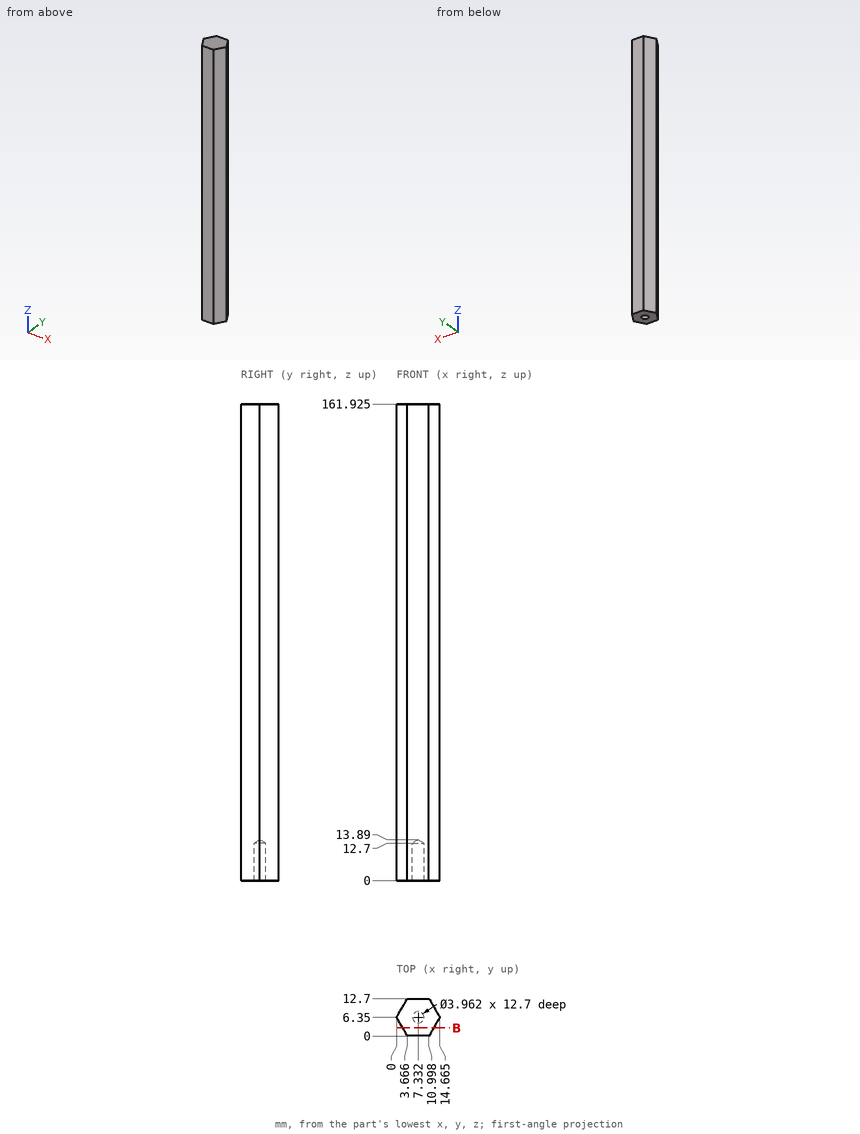
The figure shows three views and two pictorial views of one solid part (mm, origin at its lowest corner). Answer the questions. Give positions to 0.01 mm unless a question says otherwise; leave off trailing zeros. Write each loop counter-clockwise with the first axis right and the second up, starting at its lowest first coordinate (ties: lowest second). Pieces come first, ordered by that corner, then holes. Notation, with made-up numbers: M 21,70.25 L 72,70.25 A25 cw 72,83.25 Z; hole C 4.5,72.5 d5. An arc over 180 degrees is marked long. Write each question's results on one line, items separated by ' | '.
Q1. Flat-ended cylindrical pins translate along their axes: P1, Ø5, axis at y = 7, z = 51.5, coming from the -X side; P2, Ø6, axis at y = 3, z = 106.5, coming from the +X side; P3, Ø1.5, axis at y = 5.5, z = 54.5, coming from the -X side. Find the tip coordinate at first contact, or state that the pin passes through.
Output values:
P1: x = 0 | P2: x = 14.46 | P3: x = 0.06
Q2. Section B-B, the plane y = 2.75 is taken. Write down the section's boundary in (x, z) (1 decimal), then the cut area to 3 significant figures.
Output values:
outline: M 2.1,0 L 12.6,0 L 12.6,161.9 L 2.1,161.9 Z | area: 1,700 mm2
Q3. Consider L1, parallel to Y at x = 11, z = 110 (1 decimal); L2, parallel to X at y = 6, z = 11; L3, parallel to X at y = 0.5, z = 27. Determine where each line is inside the solid, lowest interval first. Write a range as from..to.
Output values:
L1: 0..12.7 | L2: 0.2..5.38, 9.28..14.46 | L3: 3.38..11.29
